Can you work these out from the drawing? Everything is in mm from the part's minimum corner. A direction names the side the tool comes from. Round coordinates to 2 decimals unless told otherwise and drop trailing zeros. Order: outer loops, then holes, each group sorted by start corner. A loop starts at its lowest first (then second) coordinate and runs counter-clockwise, first axis right, second up. Notation, with made-up numbers: M -11,59.25 L 24,59.25 A18 ccw 24,81.25 Z; hole C 5.5,10 d9. An arc over 180 degrees is marked long. Write item = value, one per line. Start each with the question number.
Item 1: Please list where these lines run through material, in increasing order: L1, parallel to X at y = 16.5, z = 2.6; L2, parallel to Y at x = 35, z = 2.2.
Item 2: I want a section at A-A, the plane z = 2.5. List the corners of the cut face in (x, y) for me.
Item 3: We'd pull the mould along Y, two halves only. Please class the marked faces 1, 2 and 3: pulls with the +Y half, pulls with the -Y half, needs draft (parallel to the pull), parting line crosses it, or undercut.
Item 4: For the marked faces 4, 5 and 6, which set-ups out of +Z, -Z, +X, -X, +Y, -Y let a thin tool reach every point of the face, with its end or its side?
Item 5: I'm going to push flat-ended pins straight in: P1, Ø1, axis at y = 0.5, z = 1.5, coming from the -X side; P2, Ø1, axis at x = 1.5, z = 2, coming from the +Y side; P3, Ø1.6, axis at y = 17, z = 2, coming from the +X side. Where does each tip first touch, or does it pass through?
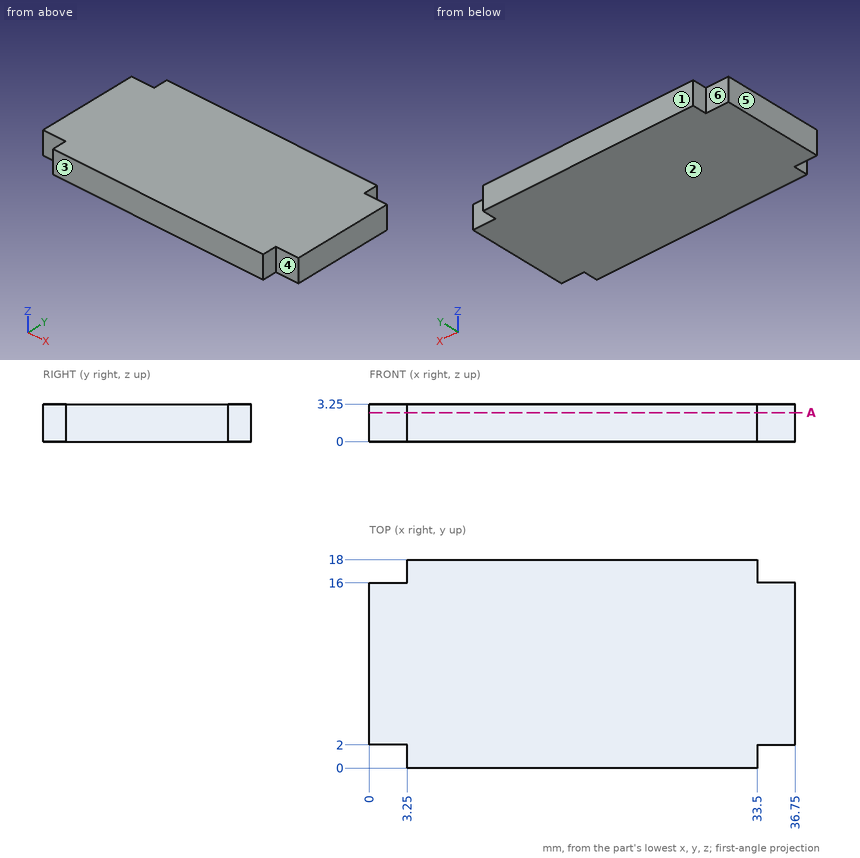
Filled in:
q1.L1 = 3.25 to 33.5
q1.L2 = 2 to 16
q2.outline = M 0,2 L 3.25,2 L 3.25,0 L 33.5,0 L 33.5,2 L 36.75,2 L 36.75,16 L 33.5,16 L 33.5,18 L 3.25,18 L 3.25,16 L 0,16 Z
q3.face_1 = pulls with the +Y half
q3.face_2 = needs draft
q3.face_3 = pulls with the -Y half
q4.face_4 = +Z, -Z, +X, -Y
q4.face_5 = +Z, -Z, -X, +Y, -Y
q4.face_6 = +Z, -Z, -X, +Y
q5.P1 = 3.25
q5.P2 = 16
q5.P3 = 33.5
